```python
from build123d import *

# Parameters (mm, degrees)
PAD_DEPTH        = 160
SKETCH001_W      = 9
SKETCH001_H      = 172.193062
POCKET_DEPTH     = 60
CHAMFER_SIZE     = 10
CHAMFER001_SIZE  = 2
HOLE_D           = 5
HOLE_CBORE_D     = 16
HOLE_CBORE_DEPTH = 22
SKETCH003_R      = 8.5
PAD001_DEPTH     = 22
CHAMFER002_SIZE  = 3


with BuildPart() as part:
    # Sketch → Pad (new body)
    with BuildSketch(Plane.XY):
        with BuildLine():
            ThreePointArc((-0.1, 23.999792), (-24, 0), (-0.1, -23.999792))
            Line((-0.1, -60), (-0.1, -23.999792))
            Line((-30.1, -60), (-0.1, -60))
            Line((-30.1, 60), (-30.1, -60))
            Line((-30.1, 60), (-0.1, 60))
            Line((-0.1, 60), (-0.1, 23.999792))
        make_face()
    extrude(amount=PAD_DEPTH)

    # Sketch001 → Pocket (cut)
    with BuildSketch(Plane.XY):
        with Locations((-4.5, 7.136196)):
            Rectangle(SKETCH001_W, SKETCH001_H)
    extrude(amount=POCKET_DEPTH, mode=Mode.SUBTRACT)

    # Chamfer
    chamfer_edges = [part.edges().sort_by_distance(p)[0] for p in [
        (-30.1, 60, 80),
        (-30.1, -60, 80),
    ]]
    chamfer(chamfer_edges, length=CHAMFER_SIZE)

    # Chamfer001
    chamfer001_edges = [part.edges().sort_by_distance(p)[0] for p in [
        (-9, -41.124298, 0),
        (-9, 41.124298, 0),
    ]]
    chamfer(chamfer001_edges, length=CHAMFER001_SIZE)

    # Hole (through all)
    with Locations(Plane(origin=(-30.1, 0, 0), x_dir=(0, -1, 0), z_dir=(-1, 0, 0))):
        with Locations((-40, 145), (-40, 75), (40, 145), (40, 75), (-40, 110), (40, 110)):
            CounterBoreHole(HOLE_D / 2, HOLE_CBORE_D / 2, HOLE_CBORE_DEPTH)

    # Sketch003 (on Face30 of Hole) → Pad001 (join)
    with BuildSketch(Plane(origin=(-8.1, 0, 0), x_dir=(0, -1, 0), z_dir=(-1, 0, 0))):
        with Locations((-40, 110)):
            Circle(SKETCH003_R)
        Polygon((-35.950555, 102.986156), (-31.90111, 110), (-35.950555, 117.013844), (-44.049445, 117.013844), (-48.09889, 110), (-44.049445, 102.986156), align=None, mode=Mode.SUBTRACT)
        with Locations((-40, 75)):
            Circle(SKETCH003_R)
        Polygon((-35.950555, 67.986156), (-31.90111, 75), (-35.950555, 82.013844), (-44.049445, 82.013844), (-48.09889, 75), (-44.049445, 67.986156), align=None, mode=Mode.SUBTRACT)
        with Locations((-40, 145)):
            Circle(SKETCH003_R)
        Polygon((-35.880447, 137.864725), (-31.760895, 145), (-35.880447, 152.135275), (-44.119553, 152.135275), (-48.239105, 145), (-44.119553, 137.864725), align=None, mode=Mode.SUBTRACT)
    extrude(amount=PAD001_DEPTH)

    # Chamfer002
    chamfer002_edges = [part.edges().sort_by_distance(p)[0] for p in [
        (-8.1, -40, 72.5),
        (-8.1, -40, 142.5),
        (-8.1, -40, 107.5),
    ]]
    chamfer(chamfer002_edges, length=CHAMFER002_SIZE)


solid = part.part
```
Model file for the job. Use its own axes, mm. A direction names the side the tool comes from. Coordinates: 2 decimals unless noted, no trailing zeros. Loops run counter-clockwise (first coordinate to the right, second up) from the corner with the lowest first, then second, coordinate; pieces in that order, holes last. Notation, with made-up numbers: (22, 6.5) -> (39, 6.5) arc R12 cw to (39, 10.5) -> close; hole circle Ø1 at (41.5, -39.75). An arc over 180 degrees is marked (long way). Answer as a JSON object with one key per item and string values.
Q1. Cut at B-B (z = 62). List the corners of the cut face in (x, y).
Report:
{"outline": "(-30.1, -50) -> (-20.1, -60) -> (-0.1, -60) -> (-0.1, -24) arc R24 cw to (-0.1, 24) -> (-0.1, 60) -> (-20.1, 60) -> (-30.1, 50) -> close"}
Q2. Probe probe 1 along Z at (x, y) = (-23.75, -40); probe 2 along Y at (x, z) = (-1.3, 145); probe 3 along Z at (x, y) = (-6, 40). List the from-to ranges inside material, lowest first.
Report:
{"probe 1": "z = 0 to 67, 83 to 102, 118 to 137, 153 to 160", "probe 2": "y = -60 to -42.5, -37.5 to -23.96, 23.96 to 37.5, 42.5 to 60", "probe 3": "z = 60 to 72.5, 77.5 to 107.5, 112.5 to 142.5, 147.5 to 160"}
Q3. Cut at D-D (z = 40). List the corners of the cut face in (x, y), and give its area (3 significant figures).
Report:
{"outline": "(-30.1, -50) -> (-20.1, -60) -> (-9, -60) -> (-9, -22.25) arc R24 cw to (-9, 22.25) -> (-9, 60) -> (-20.1, 60) -> (-30.1, 50) -> close", "area": "1,950 mm2"}
Q4. Pull direction Z, two halves, no side cores. Call faces 3 (the flat face through (-18.946, 46.205, 141.476)), 4 (the flat face through (-25, -55.1, 78.9)), 5 (the flat face through (-18.95, 46.05, 113.55)): released by +Z, released by -Z, zero draft, split by the parting line, or undercut.
Report:
{"face 3": "undercut", "face 4": "zero draft", "face 5": "undercut"}
Q5. Cut at A-A (y = 40). State how many separate pieces and enclosed holes the cut face has, and give its area (3 significant figures).
Report:
{"separate pieces": "4", "enclosed holes": "0", "area": "3,210 mm2"}
Q6. Flat gauge pins, fed straight in: P1, Ø6.5, axis at y = 40, z = 145, coming from the -X side; P2, Ø7, axis at x = -4.5, y = 33.5, coming from the -Z side. Where does each tip first touch, or does it go through?
Report:
{"P1": "stops at x = -8.1", "P2": "stops at z = 60"}
Q7. 3-axis set-ups, long thin cutter, end or side, ignore diameter. For faces 1 (the flat face through (-18.946, 33.795, 148.524)), 2 (the cylindrical face through (-4.04, 42.31, 74.04)): which of +Z, -Z, +X, -X, +Y, -Y reach the whole face in a straight line?
Report:
{"face 1": "-X", "face 2": "+X, -X"}
Q8. Cut at C-C (y = 26.5). List the corners of the cut face in (x, z), and give its area (3 significant figures).
Report:
{"outline": "(-30.1, 0) -> (-11, 0) -> (-9, 2) -> (-9, 60) -> (-0.1, 60) -> (-0.1, 160) -> (-30.1, 160) -> close", "area": "4,260 mm2"}
